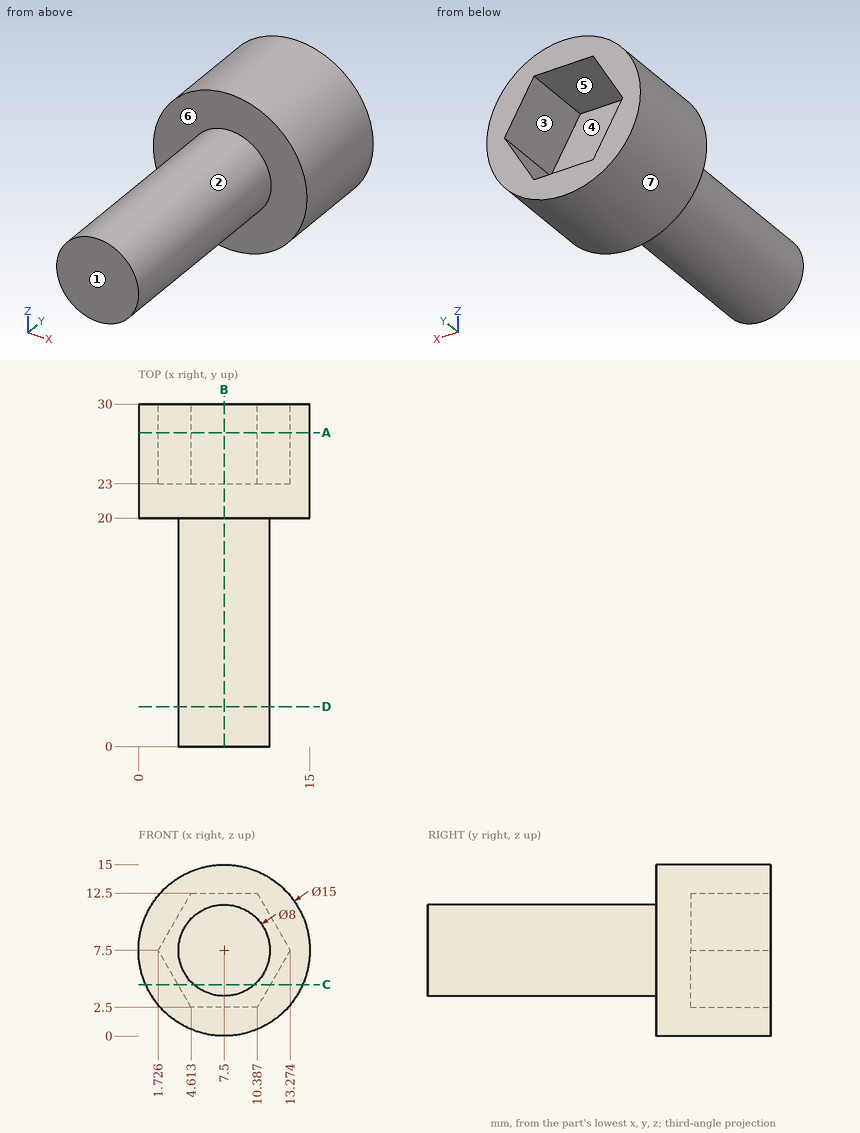
Design review of the part shown in the three views and the two pictorial views. Dimensions are in mm from the part's minimum x, y and z. A direction names the side the tool comes from. Round coordinates to 2 decimals unless told otherwise and drop trailing zeros. Loops run counter-clockwise (first coordinate to the right, second up) from the corner with the lowest first, then second, coordinate; pieces in that order, holes last. Notation, with made-up numbers: (12.5, 7.25) -> (61.5, 7.25) arc R29 ccw to (61.5, 39.25) -> close; hole circle Ø11 at (-24, 1.25). An arc over 180 degrees is marked (long way). Use one line per item in the form item = value. Start each with the question number.
Q1. Wall thickness on line 1 along Y through (x, z) = (4, 5.5); line 2 along Y through (x, z) = (9.5, 4.25); line 3 along X through (y, z) = (25.5, 4.75) (1 decimal): over which ranges is each line inside the solid? List them lowest first. Write a range as [from, to].
Q2. We need section C-C on z = 4.5. Give the boundary of the cut face in (x, y) (1 decimal).
Q3. Machinability: for the marked faces 5, 6 and 7, which of the approach directions +Z, -Z, +X, -X, +Y, -Y give a long, thin tool a straight path to every point of the face, cutting with its end or side? Answer none if there is none.
Q4. We need section D-D on y = 3.5. Give the boundary of the cut face in (x, z).
Q5. For pin 1 Ø2 at (x, z) = (2.5, 9) entering from -Y; pin 2 Ø3 at (x, y) = (12.5, 16) entering from -Z (1 decimal); pin 3 Ø5 at (y, z) = (16, 5) entering from +X, all flat-tipped, find the tip position at first contact; note any pin that passes through.
Q6. Draft analysis for pull direction Z (two halves, no side actions). For the marked faces 1, 2, 3 and 4, state which applies: +Z half, -Z half, draft (parallel to the pull), parting line (faces both ways), or undercut.
Q7. We need section B-B on x = 7.5. Give the boundary of the cut face in (y, z), then the cut area to 3 significant figures.
Q8. We need section A-A on y = 27.5. Give the boundary of the cut face in (x, z).
Calculated:
q1.line_1 = [20, 23]
q1.line_2 = [0, 23]
q1.line_3 = [0.5, 3.3], [11.7, 14.5]
q2.outline = (0.6, 20) -> (4.9, 20) -> (4.9, 0) -> (10.1, 0) -> (10.1, 20) -> (14.4, 20) -> (14.4, 30) -> (11.5, 30) -> (11.5, 23) -> (3.5, 23) -> (3.5, 30) -> (0.6, 30) -> close
q3.face_5 = +Y
q3.face_6 = -Y
q3.face_7 = +Y, -Y
q4.outline = circle Ø8 at (7.5, 7.5)
q5.pin_1 = 20
q5.pin_2 = 5.6
q5.pin_3 = 11.5
q6.face_1 = draft
q6.face_2 = parting line
q6.face_3 = undercut
q6.face_4 = undercut
q7.outline = (0, 3.5) -> (20, 3.5) -> (20, 0) -> (30, 0) -> (30, 2.5) -> (23, 2.5) -> (23, 12.5) -> (30, 12.5) -> (30, 15) -> (20, 15) -> (20, 11.5) -> (0, 11.5) -> close
q7.area = 240 mm²
q8.outline = circle Ø15 at (7.5, 7.5); hole (1.73, 7.5) -> (4.61, 2.5) -> (10.39, 2.5) -> (13.27, 7.5) -> (10.39, 12.5) -> (4.61, 12.5) -> close
